```python
from build123d import *

# Parameters (mm, degrees)
SKETCH1_R           = 7
BOSS_EXTRUDE1_DEPTH = 8
SKETCH2_OUTSIDE_W   = 21.092
SKETCH2_OUTSIDE_H   = 21.092
SKETCH2_OUTSIDE_R   = 5
CUT_EXTRUDE1_DEPTH  = 14
SKETCH3_W           = 9
SKETCH3_H           = 9.175
SKETCH4_R           = 3
CUT_EXTRUDE2_DEPTH  = 15
CUT_EXTRUDE3_DEPTH  = 9
FILLET1_R           = 1


with BuildPart() as part:
    # Sketch1 → Boss-Extrude1 (new, symmetric)
    with BuildSketch(Plane.XY):
        Circle(SKETCH1_R)
    extrude(amount=BOSS_EXTRUDE1_DEPTH, both=True)

    # Sketch2 outside → Cut-Extrude1 (cut)
    with BuildSketch(Plane(origin=(0, 0, -8), x_dir=(-1, 0, 0), z_dir=(0, 0, -1))):
        Rectangle(SKETCH2_OUTSIDE_W, SKETCH2_OUTSIDE_H)
        Circle(SKETCH2_OUTSIDE_R, mode=Mode.SUBTRACT)
    extrude(amount=-CUT_EXTRUDE1_DEPTH, mode=Mode.SUBTRACT)

    # Sketch3 → Cut-Revolve1 (revolve, cut)
    with BuildSketch(Plane(origin=(0, 0, 0), x_dir=(1, 0, 0), z_dir=(0, 1, 0)), mode=Mode.PRIVATE) as cut_revolve1_sk:
        Polygon((-5, 3.675), (-3.5, 8), (-5, 8), align=None)
        with Locations((-8.5, -1.4125)):
            Rectangle(SKETCH3_W, SKETCH3_H)
    revolve(cut_revolve1_sk.sketch.rotate(Axis((0, 0, 6), (0, 0, -1)), 180), axis=Axis((0, 0, 6), (0, 0, -1)), mode=Mode.SUBTRACT)

    # Sketch4 → Cut-Extrude2 (cut)
    with BuildSketch(Plane(origin=(0, 0, -8), x_dir=(-1, 0, 0), z_dir=(0, 0, -1))):
        Circle(SKETCH4_R)
    extrude(amount=-CUT_EXTRUDE2_DEPTH, mode=Mode.SUBTRACT)

    # Sketch5 → Cut-Extrude3 (cut)
    with BuildSketch(Plane(origin=(0, 0, -8), x_dir=(-1, 0, 0), z_dir=(0, 0, -1))):
        Polygon((-0.5, 12), (0.5, 12), (0.5, 0.5), (12, 0.5), (12, -0.5), (0.5, -0.5), (0.5, -12), (-0.5, -12), (-0.5, -0.5), (-12, -0.5), (-12, 0.5), (-0.5, 0.5), align=None)
    extrude(amount=-CUT_EXTRUDE3_DEPTH, mode=Mode.SUBTRACT)

    # Fillet1
    fillet1_edges = [part.edges().sort_by_distance(p)[0] for p in [
        (-7, 0, 8),
    ]]
    fillet(fillet1_edges, radius=FILLET1_R)


solid = part.part
```
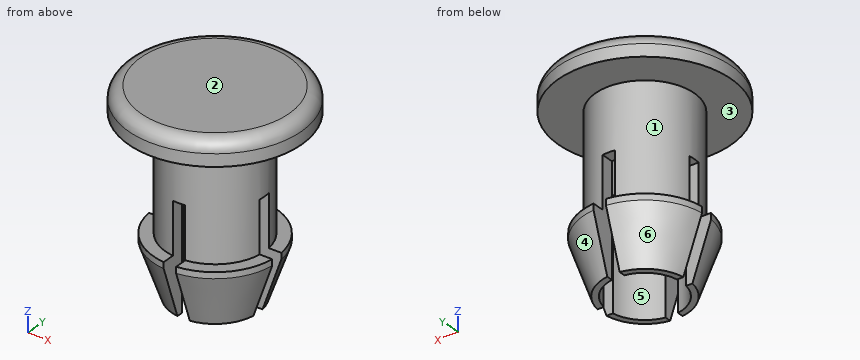
Model file for the job. Use its own axes, mm. Face numbers are marked on the shaded views. A direction names the side the tool comes from. Coordinates: 2 decimals unless noted, no trailing zeros. Loops run counter-clockwise (first coordinate to the right, second up) from the corner with the lowest first, then second, coordinate; pieces in that order, holes last. Notation, with made-up numbers: (14.5, 37.25) - (33.5, 37.25) arc R13 ccw to (33.5, 41.25) - close; hole circle Ø7 at (63, -3.75). An arc over 180 degrees is marked (long way). Answer as a JSON object with one key per item and string values. Group by question number.
(1) Flat gauge pins, fed straight in: pin 1 (0.6 mm diameter, centred on y = -3.5, z = -3, fed in from +X); pin 2 (0.5 mm diameter, centred on x = 3.5, y = 0, fed in from -Z); pin 3 (0.6 mm diameter, centred on x = 4, z = -2.5, fed in from -Y). Where does each tip first touch, or does it go through?
(2) Tool access for the marked faces 5 and 6: list every direction of +Z, -Z, +X, -X, +Y, -Y with a clear straight run to the whole face (end or side of a thin tool).
(3) Cut at D-D (z = -5.75). Give the cut face in (x, y).
(4) Cut at A-A (y = 0). Give the cut face in (x, z), then the cut area to 3 significant figures.
(5) Two-plate mould, pull along Z, no slides. Class the marked faces 1, 2, 3 and 4: released by +Z, released by -Z, zero draft, split by the parting line, or undercut.
(6) Cut at B-B (z = 6.25). Give the cut face in (x, y), then the cut area to 3 significant figures.
(7) Probe line 1 along Y through (x, z) = (0, 2.5); line 2 along Z through (x, y) = (-5, -3); line 3 along Z through (x, y) = (2.25, 1.25). List the from-to ranges inside material, lowest first.
Geometry says:
{
 "1": {"pin 1": "stops at x = 3.79", "pin 2": "stops at z = 1", "pin 3": "stops at y = -1.52"},
 "2": {"face 5": "-Z", "face 6": "-Z, -X, +Y"},
 "3": {"outline": "(-4.25, -0.5) arc R4.28 ccw to (-0.5, -4.25) - (-0.5, -2.96) arc R3 cw to (-2.96, -0.5) - close; (-4.25, 0.5) - (-2.96, 0.5) arc R3 cw to (-0.5, 2.96) - (-0.5, 4.25) arc R4.28 ccw to start; (0.5, -4.25) arc R4.28 ccw to (4.25, -0.5) - (2.96, -0.5) arc R3 cw to (0.5, -2.96) - close; (0.5, 2.96) arc R3 cw to (2.96, 0.5) - (4.25, 0.5) arc R4.28 ccw to (0.5, 4.25) - close"},
 "4": {"outline": "(-7, 6) - (-4, 6) - (-4, 1) - (-3, 1) - (-3, 7) - (3, 7) - (3, 1) - (4, 1) - (4, 6) - (7, 6) - (7, 7) arc R1 ccw to (6, 8) - (-6, 8) arc R1 ccw to (-7, 7) - close", "area": "31.6 mm^2"},
 "5": {"face 1": "undercut", "face 2": "released by +Z", "face 3": "undercut", "face 4": "released by -Z"},
 "6": {"outline": "circle Ø14 at (0, 0); hole circle Ø6 at (0, 0)", "area": "126 mm^2"},
 "7": {"line 1": "y = -4 to -3, 3 to 4", "line 2": "z = 6 to 8", "line 3": "z = 7 to 8"}
}
